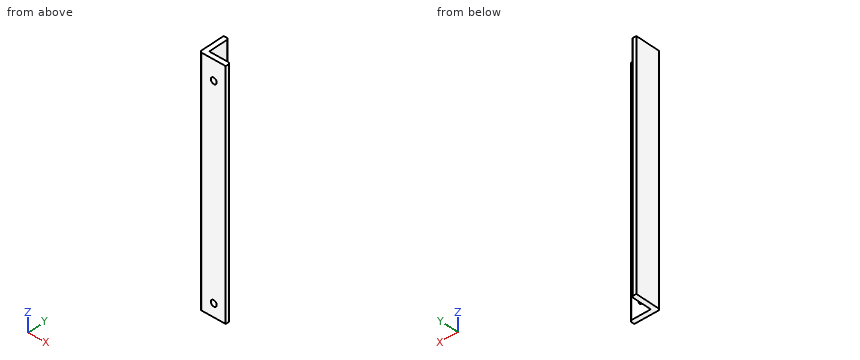
Autodesk Inventor part; units mm, degrees
ref_plane "YZ Plane" through (0, 0, 0) normal (1, 0, 0) x (0, 1, 0)
ref_plane "XZ Plane" through (0, 0, 0) normal (0, 1, 0) x (-1, 0, 0)
ref_plane "XY Plane" through (0, 0, 0) normal (0, 0, 1) x (1, 0, 0)
sketch "Sketch1" plane through (0, 0, 0) normal (0, 0, 1) x (1, 0, 0)
  line L0 (52.418, 170.3116) -> (67.15, 170.3116)
  line L1 (67.15, 170.3116) -> (67.15, 167.2636)
  line L2 (51.148, 171.5816) -> (51.148, 186.3136)
  line L3 (51.148, 186.3136) -> (52.926, 186.3136)
  line L4 (54.196, 185.0436) -> (54.196, 173.3596)
  line L5 (67.15, 170.3116) -> (67.15, 172.0896)
  line L6 (65.88, 173.3596) -> (54.196, 173.3596)
  arc A0 (54.196, 185.0436) -> (52.926, 186.3136) centre (52.926, 185.0436) ccw
  arc A1 (67.15, 172.0896) -> (65.88, 173.3596) centre (65.88, 172.0896) ccw
  arc A2 (51.148, 171.5816) -> (52.418, 170.3116) centre (52.418, 171.5816) ccw
  point P0 (0, 0)
  point P1 (51.148, 170.3116)
  point P2 (54.196, 186.3136)
  point P3 (67.15, 173.3596)
  dimension "d0" = 16.002
  dimension "d1" = 3.048
  dimension "d2" = 16.002
  dimension "d3" = 3.048
  dimension "d4" = 3.048
  dimension "d5" = 1.27
  dimension "d6" = 1.27
extrude "Extrusion1" add sketch "Sketch1" along normal blind 146.304
sketch "Sketch3" plane through (54.196, 173.3596, 0) normal (0, 1, 0) x (1, 0, 0)
  line L0 (0.9375, 6.2475) -> (13.2819, 6.2475)
  line L1 (12.954, 0) -> (-1.778, 0)
  line L2 (5.588, 0) -> (5.588, -6.1341)
  line L3 (-1.778, -146.304) -> (12.954, -146.304)
  circle A0 centre (5.588, -7.9756) radius 1.8415
  line L4 (5.588, -7.9756) -> (5.588, -130.5306)
  circle A1 centre (5.588, -134.2136) radius 1.8415
  point P0 (-54.196, 0)
  dimension "d31" = 12.3444
  dimension "d32" = 6.1341
  dimension "d38" = 122.555
extrude "Extrusion6" cut sketch "Sketch3" against normal blind 69.85
CAD build for the part. Positions are in the model's coordinates, mm. Round coordinates to 2 decimals unless told otherwise and drop trailing zeros. Order: outer loops, then holes, each group sorted by start corner. A loop starts at its lowest first (then second) coordinate and runs counter-clockwise, first axis right, second up. Notation, with made-up numbers: (72.25, 65.5) - (121.25, 65.5) arc R31 cw to (121.25, 91.5) - close; hole circle Ø8 at (50, 7.5). An arc over 180 degrees is marked (long way). Answer in a Markdown table with one row per item. Add a question column.
(1) Band-saw the part on A-A on z = 120. List the corners of the cut face in (x, y).
(2) Drop flat-ended pins along their axis: pin 1 Ø2 at (x, y) = (57.5, 175.5) entering from -Z; pin 2 Ø3 at (y, z) = (181.5, 63) entering from +X; pin 3 Ø6 at (x, z) = (61, 65.5) entering from +Y. Give the stop position or say it passes through.
(3) Probe L1, parallel to X at y = 174.25, z = 84.5; L2, parallel to Y at x = 55.75, z = 63.5; L3, parallel to X at y = 172.25, z = 80. List the from-to ranges inside material, lowest first. Write a range as [from, to].
(4) Band-saw the part on B-B on y = 179.5. List the corners of the cut face in (x, z), and give its area (3 significant figures).
Data:
| question | item | result |
|---|---|---|
| 1 | outline | (51.15, 171.58) arc R1.27 ccw to (52.42, 170.31) - (67.15, 170.31) - (67.15, 172.09) arc R1.27 ccw to (65.88, 173.36) - (54.2, 173.36) - (54.2, 185.04) arc R1.27 ccw to (52.93, 186.31) - (51.15, 186.31) - close |
| 2 | pin 1 | passes through |
| 2 | pin 2 | stops at x = 54.2 |
| 2 | pin 3 | stops at y = 173.36 |
| 3 | L1 | x = [51.15, 54.2] |
| 3 | L2 | y = [170.31, 173.36] |
| 3 | L3 | x = [51.15, 67.14] |
| 4 | outline | (51.15, 0) - (54.2, 0) - (54.2, 146.3) - (51.15, 146.3) - close |
| 4 | area | 446 mm^2 |
